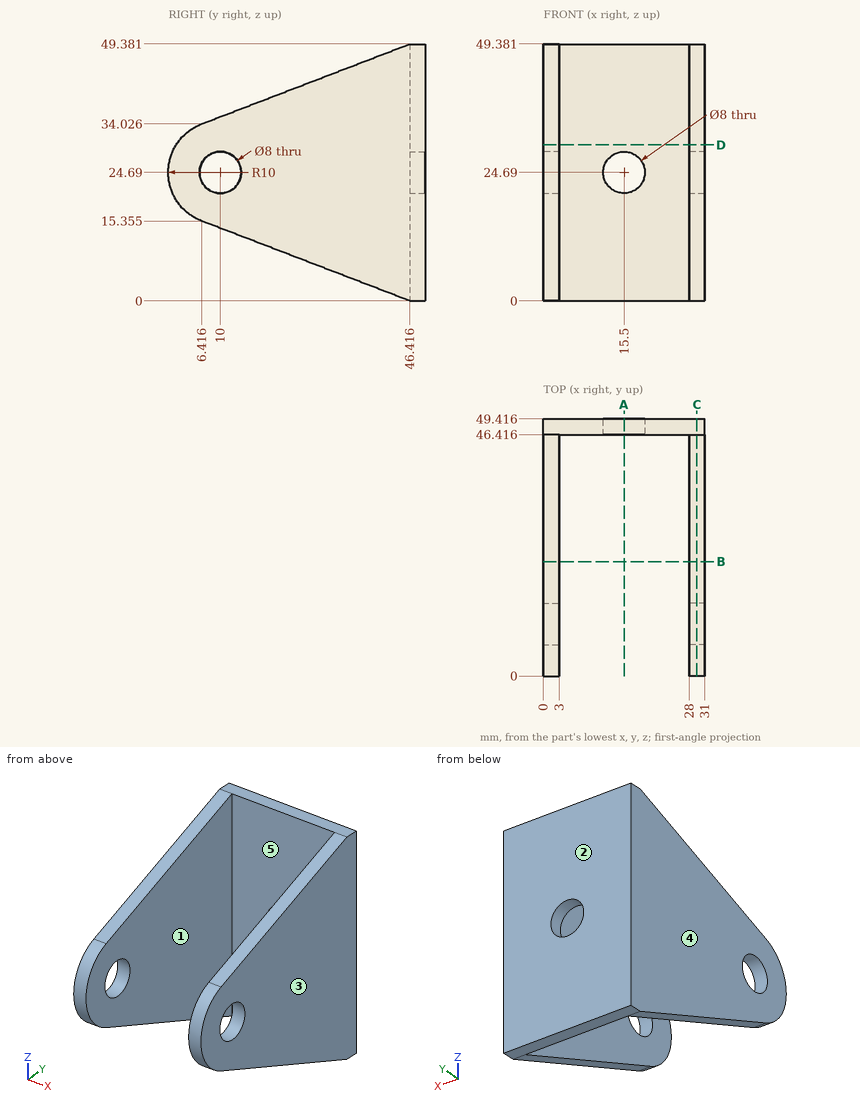
Source: three-view drawing plus pictorial views. Frame: mm from the lowest corner of the part. A direction names the side the tool comes from. Round coordinates to 2 decimals unless told otherwise and drop trailing zeros. Loops run counter-clockwise (first coordinate to the right, second up) from the corner with the lowest first, then second, coordinate; pieces in that order, holes last. Notation, with made-up numbers: M 80.5,22 L 123.5,22 A25 ccw 123.5,36 Z; hole C 23,22.5 d2. An arc over 180 degrees is marked long. Put each result on its own line as item: value.
(1) Access query for the marked faces 4 and 5. Directions: +Z, -Z, +X, -X, +Y, -Y. A direction counts if a zero-diameter tool reaches every point of the face in a straight line with its end or side. Return the directions, or none.
Solutions:
face 4: +Z, -Z, -X, +Y, -Y
face 5: +Z, -Z, -Y
(2) Pull-direction query (X, two-part tool) for the marked faces 1, 2 and 3; classes: released by +X, released by -X, zero draft, split by the parting line, or undercut.
Solutions:
face 1: undercut
face 2: zero draft
face 3: released by +X
(3) First-contact query: pin 1 (1 mm diameter, centred on x = 15, z = 42.5, fed in from -Y); pin 2 (5 mm diameter, centred on y = 10, z = 24.69, fed in from -X); pin 3 (4 mm diameter, centred on x = 4.5, z = 17.5, fed in from -Y). Flat tips, straight axial feed; report the tip coordinate or a pass-through.
Solutions:
pin 1: y = 46.42
pin 2: through
pin 3: y = 1.9
(4) Ray query, line 1 (X direction, y = 6.5, z = 33); line 2 (Y direction, x = 3.5, z = 18); line 3 (Z direction, x = 15.5, y = 47.75). Return the intervals inside material, ascending. Write a range as [from, to].
Solutions:
line 1: [0, 3], [28, 31]
line 2: [46.42, 49.42]
line 3: [0, 20.69], [28.69, 49.38]
(5) Section D-D, the plane z = 30. Return loops of the section in (x, y).
Solutions:
outline: M 0,1.53 L 3,1.53 L 3,46.42 L 28,46.42 L 28,1.53 L 31,1.53 L 31,49.42 L 0,49.42 Z
(6) Section C-C, the plane x = 29.5. Return loops of the section in (y, z) (1 decimal).
Solutions:
outline: M 6.4,15.4 L 46.4,0 L 49.4,0 L 49.4,49.4 L 46.4,49.4 L 6.4,34 A10 ccw Z; hole C 10,24.7 d8
(7) Section A-A, the plane x = 15.5. Return loops of the section in (y, z), and give its area (3 significant figures).
Solutions:
outline: M 46.42,0 L 49.42,0 L 49.42,20.69 L 46.42,20.69 Z; M 46.42,28.69 L 49.42,28.69 L 49.42,49.38 L 46.42,49.38 Z
area: 124 mm²
(8) Section B-B, the plane y = 22. Return loops of the section in (x, z), and give its area (3 significant figures).
Solutions:
outline: M 0,9.37 L 3,9.37 L 3,40.01 L 0,40.01 Z; M 28,9.37 L 31,9.37 L 31,40.01 L 28,40.01 Z
area: 184 mm²
